from build123d import *

# Parameters (mm, degrees)
F1_R     = 100
F2_DEPTH = 25
F0_R     = 5
F3_DEPTH = 25.001


with BuildPart() as f2:
    # F1 (on Top) → F2 (new body)
    with BuildSketch(Plane.XY):
        Circle(F1_R)
    extrude(amount=F2_DEPTH)

    # F0 (on Top) → F3 (cut, through all)
    with BuildSketch(Plane.XY):
        Circle(F0_R)
        with Locations((0, 20)):
            Circle(F0_R)
        with Locations((0, 40)):
            Circle(F0_R)
        with Locations((0, 60)):
            Circle(F0_R)
        with Locations((0, 80)):
            Circle(F0_R)
        with Locations((-20.705524, 77.274066)):
            Circle(F0_R)
        with Locations((-40, 69.282032)):
            Circle(F0_R)
        with Locations((-56.568542, 56.568542)):
            Circle(F0_R)
        with Locations((-69.282032, 40)):
            Circle(F0_R)
        with Locations((-77.274066, 20.705524)):
            Circle(F0_R)
        with Locations((-80, 0)):
            Circle(F0_R)
        with Locations((-77.274066, -20.705524)):
            Circle(F0_R)
        with Locations((-69.282032, -40)):
            Circle(F0_R)
        with Locations((-56.568542, -56.568542)):
            Circle(F0_R)
        with Locations((-40, -69.282032)):
            Circle(F0_R)
        with Locations((-20.705524, -77.274066)):
            Circle(F0_R)
        with Locations((0, -80)):
            Circle(F0_R)
        with Locations((20.705524, -77.274066)):
            Circle(F0_R)
        with Locations((40, -69.282032)):
            Circle(F0_R)
        with Locations((56.568542, -56.568542)):
            Circle(F0_R)
        with Locations((69.282032, -40)):
            Circle(F0_R)
        with Locations((77.274066, -20.705524)):
            Circle(F0_R)
        with Locations((80, 0)):
            Circle(F0_R)
        with Locations((77.274066, 20.705524)):
            Circle(F0_R)
        with Locations((69.282032, 40)):
            Circle(F0_R)
        with Locations((56.568542, 56.568542)):
            Circle(F0_R)
        with Locations((40, 69.282032)):
            Circle(F0_R)
        with Locations((20.705524, 77.274066)):
            Circle(F0_R)
        with Locations((-17.68531, 57.334368)):
            Circle(F0_R)
        with Locations((-33.799203, 49.574326)):
            Circle(F0_R)
        with Locations((-46.909889, 37.409388)):
            Circle(F0_R)
        with Locations((-55.852425, 21.920461)):
            Circle(F0_R)
        with Locations((-59.832228, 4.483806)):
            Circle(F0_R)
        with Locations((-58.495675, -13.351256)):
            Circle(F0_R)
        with Locations((-51.961524, -30)):
            Circle(F0_R)
        with Locations((-40.810364, -43.983112)):
            Circle(F0_R)
        with Locations((-26.033024, -54.058132)):
            Circle(F0_R)
        with Locations((-8.942536, -59.32985)):
            Circle(F0_R)
        with Locations((8.942536, -59.32985)):
            Circle(F0_R)
        with Locations((26.033024, -54.058132)):
            Circle(F0_R)
        with Locations((40.810364, -43.983112)):
            Circle(F0_R)
        with Locations((51.961524, -30)):
            Circle(F0_R)
        with Locations((58.495675, -13.351256)):
            Circle(F0_R)
        with Locations((59.832228, 4.483806)):
            Circle(F0_R)
        with Locations((55.852425, 21.920461)):
            Circle(F0_R)
        with Locations((46.909889, 37.409388)):
            Circle(F0_R)
        with Locations((33.799203, 49.574326)):
            Circle(F0_R)
        with Locations((17.68531, 57.334368)):
            Circle(F0_R)
        with Locations((-15.63663, 12.469796)):
            Circle(F0_R)
        with Locations((-19.498558, -4.450419)):
            Circle(F0_R)
        with Locations((-8.677675, -18.019377)):
            Circle(F0_R)
        with Locations((8.677675, -18.019377)):
            Circle(F0_R)
        with Locations((19.498558, -4.450419)):
            Circle(F0_R)
        with Locations((15.63663, 12.469796)):
            Circle(F0_R)
        with Locations((-17.35535, 36.038755)):
            Circle(F0_R)
        with Locations((-31.273259, 24.939592)):
            Circle(F0_R)
        with Locations((-38.997116, 8.900837)):
            Circle(F0_R)
        with Locations((-38.997116, -8.900837)):
            Circle(F0_R)
        with Locations((-31.273259, -24.939592)):
            Circle(F0_R)
        with Locations((-17.35535, -36.038755)):
            Circle(F0_R)
        with Locations((0, -40)):
            Circle(F0_R)
        with Locations((17.35535, -36.038755)):
            Circle(F0_R)
        with Locations((31.273259, -24.939592)):
            Circle(F0_R)
        with Locations((38.997116, -8.900837)):
            Circle(F0_R)
        with Locations((38.997116, 8.900837)):
            Circle(F0_R)
        with Locations((31.273259, 24.939592)):
            Circle(F0_R)
        with Locations((17.35535, 36.038755)):
            Circle(F0_R)
    extrude(amount=F3_DEPTH, mode=Mode.SUBTRACT)


solid = f2.part
Design review of the part built by this model. Coordinates are the model's own, in mm. Coordinates: 2 decimals unless noted, no trailing zeros. Order: outer loops, then holes, each group sorted by start corner. A loop starts at its lowest first (then second) coordinate and runs counter-clockwise, first axis right, second up. Notation, with made-up numbers: (-3, 65.25) - (1, 65.25) arc R9 cw to (1, 72.25) - close; hole circle Ø1 at (8, 12.25). An arc over 180 degrees is marked (long way). Put each result on its own line as item: value.
1) Insertion check: P1, Ø6, axis at x = -40, y = 69.28, coming from the +Z side; P2, Ø2, axis at x = 5, z = 9.5, coming from the +Y side; P3, Ø3, axis at y = -8, z = 11.5, coming from the +X side; P4, Ø12, axis at y = -12.5, z = 13.5, coming from the -X side. Each pin has a flat end and moves straight along its axis. Give the tip position at first contact, or say it passes through.
Response values:
P1: passes through
P2: stops at y = 99.92
P3: stops at x = 99.79
P4: stops at x = -99.79
2) Take a section at B-B, the plane z = 16. Count the separate pieces of the cut face and the enclosed holes in it, and give its area (3 significant figures).
Response values:
separate pieces: 1
enclosed holes: 67
area: 26,200 mm²
3) Take a section at A-A, the plane y = 80. Give the boundary of the cut face in (x, z).
Response values:
outline: (-60, 0) - (-24.9, 0) - (-24.9, 25) - (-60, 25) - close; (-16.51, 0) - (-5, 0) - (-5, 25) - (-16.51, 25) - close; (5, 0) - (16.51, 0) - (16.51, 25) - (5, 25) - close; (24.9, 0) - (60, 0) - (60, 25) - (24.9, 25) - close
4) Wall thickness on L1, parallel to X at y = -10.5, z = 17.75; L2, parallel to X at y = 42, z = 11.75; L3, parallel to Y at x = 78, z = 10: over which ranges is each line inside the solid? List them lowest first. Write a range as from..to.
Response values:
L1: x = -99.45..-62.6, -54.39..-43.73, -34.26..34.26, 43.73..54.39, 62.6..99.45
L2: x = -90.75..-73.86, -64.7..-48.89, -44.93..-4.58, 4.58..44.93, 48.89..64.7, 73.86..90.75
L3: y = -62.58..-25.65, -15.76..-4.58, 4.58..15.76, 25.65..62.58
